from build123d import *

# Parameters (mm, degrees)
SKETCH1_W                = 32
SKETCH1_H                = 38
SKETCH1_R                = 2
BOSS_EXTRUDE1_DEPTH      = 1.5
BOSS_EXTRUDE2_DEPTH      = 6.5
BOSS_EXTRUDE2_DEPTH_BACK = 6.5
SKETCH2_R                = 15


with BuildPart() as part:
    # Sketch1 → Boss-Extrude1 (new body)
    with BuildSketch(Plane(origin=(0, 0, 0), x_dir=(1, 0, 0), z_dir=(0, 1, 0))):
        with Locations((3.177060701, -4.044161192)):
            Rectangle(SKETCH1_W, SKETCH1_H)
        with Locations(Location((-8.822939299, 10.955838808, 0), (0, 0, 270))):
            Circle(SKETCH1_R, mode=Mode.SUBTRACT)
        with Locations(Location((15.177060701, 10.955838808, 0), (0, 0, 270))):
            Circle(SKETCH1_R, mode=Mode.SUBTRACT)
        with Locations(Location((15.177060701, -19.044161192, 0), (0, 0, 270))):
            Circle(SKETCH1_R, mode=Mode.SUBTRACT)
        with Locations(Location((-8.33660746, -19.044161192, 0), (0, 0, 270))):
            Circle(SKETCH1_R, mode=Mode.SUBTRACT)
    extrude(amount=-BOSS_EXTRUDE1_DEPTH)

    # Sketch2 → Boss-Extrude2 (add, two sides: drawn at the far end of the back side and taken through both)
    with BuildSketch(Plane.ZY.offset(-3.177060701).offset(-BOSS_EXTRUDE2_DEPTH_BACK)):
        with Locations((-9.466353074, -27)):
            Circle(SKETCH2_R)
        with BuildLine():
            Line((13.494241004, -1.5), (-9.466353074, -1.5))
            Line((-9.466353074, -1.5), (-9.466353074, -12))
            ThreePointArc((-9.466353074, -12), (-0.375906326, -15.068370693), (4.99549237, -23.018162943))
            Line((4.99549237, -23.018162943), (13.494241004, -1.5))
        make_face()
    extrude(amount=BOSS_EXTRUDE2_DEPTH + BOSS_EXTRUDE2_DEPTH_BACK)


solid = part.part
Part model, mm, in its own coordinate system. A direction names the side the tool comes from. Give positions to 0.01 mm unless a question says otherwise; leave off trailing zeros. Loops run counter-clockwise (first coordinate to the right, second up) from the corner with the lowest first, then second, coordinate; pieces in that order, holes last. Notation, with made-up numbers: M -32.5,-1 L -24.5,-1 A27 ccw -24.5,25 Z; hole C -26,-29 d11. An arc over 180 degrees is marked long. Put each result on its own line as item: value. Start each with the question number.
1) Probe probe 1 along X at (y, z) = (-24, -5.5); probe 2 along Y at (x, z) = (-4, 0.5); probe 3 along Y at (x, z) = (4, -9). List the from-to ranges inside material, lowest first.
2) 3-axis set-ups, long thin cutter, end or side, ignore diameter. For faces 1 (the flat face through (-3.323, -21, -6)), 2 (the flat face through (3, -1, 23.044)), 3 (the flat face through (9.677, -21, -6)), 4 (the flat face through (19.177, -1, 4)), 5 (the flat face through (3, -7, -9.466)): which of +Z, -Z, +X, -X, +Y, -Y reach the whole face in a straight line?
3) Saw through at C-C (x = -4). List the corners of the cut face in (y, z).
4) Pull direction Z, two halves, no side cores. Call faces 6 (the flat face through (3, 0, 4)), 7 (the cylindrical face through (3.268, -38.607, -18.967)), 8 (the cylindrical face through (-10.04, -0.74, -12.543)), 9 (the flat face through (3, -1, -14.956)): +Z half, -Z half, draft (parallel to the pull), parting line (faces both ways), or undercut.
5) Flat gauge pins, fed straight in: pin 1 (5 mm diameter, centred on x = 0.5, y = -7.5, fed in from -Z); pin 2 (4 mm diameter, centred on x = 15, z = 13.5, fed in from -Y); pin 3 (16 mm diameter, centred on x = 5, z = 5.5, fed in from -Y). Where does each tip first touch, or does it go through?
6) Saw through at A-A (z = 2). List the corners of the cut face in (x, y).
7) Saw through at B-B (y = -27). List the corners of the cut face in (x, z), then the cut area to 3 significant figures.
Numbers:
1. probe 1: -3.32 to 9.68
1. probe 2: -1.5 to 0
1. probe 3: -41.99 to 0
2. face 1: +Z, -Z, -X, -Y
2. face 2: +Z, +X, -X, +Y, -Y
2. face 3: +Z, -Z, +X, -Y
2. face 4: +Z, -Z, +X, +Y, -Y
2. face 5: -Z, +X, -X
3. outline: M -1.5,-14.96 L 0,-14.96 L 0,23.04 L -1.5,23.04 Z
4. face 6: draft
4. face 7: parting line
4. face 8: undercut
4. face 9: -Z half
5. pin 1: z = -9.47
5. pin 2: y = -1.5
5. pin 3: y = -40.28
6. outline: M -12.82,-1.5 L -3.32,-1.5 L -3.32,-36.67 L 9.68,-36.67 L 9.68,-1.5 L 19.18,-1.5 L 19.18,0 L -12.82,0 Z
7. outline: M -3.32,-24.47 L 9.68,-24.47 L 9.68,5.53 L -3.32,5.53 Z
7. area: 390 mm^2
